```python
from build123d import *

# Parameters (mm, degrees)
SKETCH1_W                          = 8.4328
SKETCH1_H                          = 7.9375
F_5_16_24_TAPPED_HOLE1_D           = 7.9375
F_5_16_24_TAPPED_HOLE1_DEPTH       = 8.4328
F_5_16_24_TAPPED_HOLE1_CSINK_D     = 9.2075
F_5_16_24_TAPPED_HOLE1_CSINK_ANGLE = 120
SKETCH4_W                          = 18.873319712
SKETCH4_H                          = 3.5052
FILLET1_R                          = 0.254
F_6_32_TAPPED_HOLE1_D              = 3.5052
F_6_32_TAPPED_HOLE1_DEPTH          = 3.5062
CIRPATTERN1_COUNT                  = 4
CHAMFER1_SIZE                      = 0.635


with BuildPart() as part:
    # Sketch1 → Base-Revolve (revolve)
    with BuildSketch(Plane(origin=(0, 0, 0), x_dir=(0, 1, 0), z_dir=(0, 0, 1)), mode=Mode.PRIVATE) as base_revolve_sk:
        with Locations((-1.2446, 3.96875)):
            Rectangle(SKETCH1_W, SKETCH1_H)
    revolve(base_revolve_sk.sketch.rotate(Axis((0, -5.461, 0), (0, 1, 0)), 180), axis=Axis((0, -5.461, 0), (0, 1, 0)))  # turned: the seam where the file's is

    # 5_16-24 Tapped Hole1
    with Locations(Plane(origin=(0, 2.9718, 0), x_dir=(-1, 0, 0), z_dir=(0, 1, 0))):
        with Locations((0, 0)):
            CounterSinkHole(F_5_16_24_TAPPED_HOLE1_D / 2, F_5_16_24_TAPPED_HOLE1_CSINK_D / 2, depth=F_5_16_24_TAPPED_HOLE1_DEPTH, counter_sink_angle=F_5_16_24_TAPPED_HOLE1_CSINK_ANGLE)

    # Sketch4 → Revolve1 (revolve)
    with BuildSketch(Plane.XY, mode=Mode.PRIVATE) as revolve1_sk:
        with Locations((-9.436659856, -7.2136)):
            Rectangle(SKETCH4_W, SKETCH4_H)
    revolve(revolve1_sk.sketch.rotate(Axis((0, -29.193959905, 0), (0, 1, 0)), 180), axis=Axis((0, -29.193959905, 0), (0, 1, 0)))  # turned: the seam where the file's is

    # Sketch5 → 5_16-18 Tapped Hole2 (revolve, cut)
    with BuildSketch(Plane(origin=(0, -5.461, 0), x_dir=(0, 0, 1), z_dir=(1, 0, 0))):
        Polygon((0, 0), (0, 3.5052), (4.60375, 3.5052), (3.96875, 3.138582579), (3.96875, 0), align=None)
    revolve(axis=Axis((0, 0.889, 0), (0, -1, 0)), mode=Mode.SUBTRACT)

    # Fillet1
    fillet1_edges = [part.edges().sort_by_distance(p)[0] for p in [
        (-7.9375, -5.461, 0),
    ]]
    fillet(fillet1_edges, radius=FILLET1_R)

    # 6-32 Tapped Hole1
    with Locations(Plane.XZ.offset(8.9662)):
        with Locations((0, 12.7)):
            f_6_32_tapped_hole1 = Hole(F_6_32_TAPPED_HOLE1_D / 2, depth=F_6_32_TAPPED_HOLE1_DEPTH)

    # CirPattern1: 6-32 Tapped Hole1 ×4 about axis
    cirpattern1_axis = Axis((0, 0, 0), (0, 1, 0))
    for i in range(1, CIRPATTERN1_COUNT):
        add(f_6_32_tapped_hole1.rotate(cirpattern1_axis, i * 360 / CIRPATTERN1_COUNT), mode=Mode.SUBTRACT)

    # Chamfer1
    chamfer1_edges = [part.edges().sort_by_distance(p)[0] for p in [
        (-18.873319712, -5.461, 0),
    ]]
    chamfer(chamfer1_edges, length=CHAMFER1_SIZE)


solid = part.part
```
The listing builds one solid part. Answer for the finished solid, in the listing's coordinates (mm). A direction names the side the tool comes from. Give positions to 0.01 mm unless a question says otherwise; leave off trailing zeros. Order: outer loops, then holes, each group sorted by start corner. A loop starts at its lowest first (then second) coordinate and runs counter-clockwise, first axis right, second up. Notation, with made-up numbers: (88, 27.5) - (135, 27.5) arc R15 ccw to (135, 37.5) - close; hole circle Ø2 at (26, 85). An arc over 180 degrees is marked (long way). Answer in a Markdown table with one row per item. Add a question column.
Q1. Given P1, Ø5, axis at y = -7.5, z = -4, coming from the -X side; P2, Ø1, axis at x = 8, y = -7, coming from the +Z side; P3, Ø5.5, axis at x = 0, z = -12.7, coming from the +Y side, each flat-ended and moving along its own axis, determine where each tip first touches the part or whether it passes through.
Q2. The part is cut by section D-D (y = -3.5). Determine the outline of the cut face in (x, z) (1 decimal).
Q3. Find the intervals of material crossed by line 1 along Z through (x, y) = (0, -7); line 2 along Z through (x, y) = (0, 1); line 3 along Y through (x, z) = (7, -6.5), in increasing order. Write a range as [from, to].
Q4. The part is cut by section A-A (x = 0). Determine the outline of the cut face in (y, z), then the cut area to 3 significant figures.
Q5. For a pull along Z with two mould halves and no side action, classify faces 1 (the cylindrical face through (0.38, -7.19, 10.99)), 2 (the flat face through (4, -8.966, 4)), 3 (the cylindrical face through (-2.457, -7.511, -18.713)), 4 (the cylindrical face through (10.99, -7.19, -0.38)) as released by +Z, released by -Z, zero draft, split by the parting line, or undercut.
Q6. The part is cut by section C-C (y = -7.5). Determine the outline of the cut face in (x, z), then the cut area to 3 significant figures.
Q7. Which of the six approach directions +Z, -Z, +X, -X, +Y, -Y give full straight-line access (tool end or side, diameter ignored) to faces 5 (the cylindrical face through (-0.38, -7.19, -10.99)), 6 (the cylindrical face through (-1.72, -1.06, 7.75))?
Q8. The part is cut by section B-B (z = 0). Determine the outline of the cut face in (x, y), then the cut area to 3 significant figures.
Determined:
| question | item | result |
|---|---|---|
| 1 | P1 | stops at x = -18.81 |
| 1 | P2 | stops at z = 17.32 |
| 1 | P3 | stops at y = -5.46 |
| 2 | outline | circle Ø15.9 at (0, 0); hole circle Ø7.9 at (0, 0) |
| 3 | line 1 | z = [-18.87, -14.45], [-10.95, -3.97], [3.97, 10.95], [14.45, 18.87] |
| 3 | line 2 | z = [-7.94, -3.97], [3.97, 7.94] |
| 3 | line 3 | y = [-8.97, -5.46] |
| 4 | outline | (-8.97, -18.87) - (-6.1, -18.87) - (-5.46, -18.24) - (-5.46, -14.45) - (-8.97, -14.45) - close; (-8.97, -10.95) - (-5.46, -10.95) - (-5.46, -8.19) arc R0.25 cw to (-5.21, -7.94) - (2.97, -7.94) - (2.97, -4.6) - (2.61, -3.97) - (-8.6, -3.97) - (-8.97, -4.6) - close; (-8.97, 4.6) - (-8.6, 3.97) - (2.61, 3.97) - (2.97, 4.6) - (2.97, 7.94) - (-5.21, 7.94) arc R0.25 cw to (-5.46, 8.19) - (-5.46, 10.95) - (-8.97, 10.95) - close; (-8.97, 14.45) - (-5.46, 14.45) - (-5.46, 18.24) - (-6.1, 18.87) - (-8.97, 18.87) - close |
| 4 | area | 146 mm² |
| 5 | face 1 | undercut |
| 5 | face 2 | zero draft |
| 5 | face 3 | split by the parting line |
| 5 | face 4 | undercut |
| 6 | outline | circle Ø37.75 at (0, 0); hole circle Ø3.51 at (-12.7, 0); hole circle Ø7.94 at (0, 0); hole circle Ø3.51 at (0, -12.7); hole circle Ø3.51 at (0, 12.7); hole circle Ø3.51 at (12.7, 0) |
| 6 | area | 1,030 mm² |
| 7 | face 5 | +Y, -Y |
| 7 | face 6 | +Y |
| 8 | outline | (-18.87, -8.97) - (-14.45, -8.97) - (-14.45, -5.46) - (-18.24, -5.46) - (-18.87, -6.1) - close; (-10.95, -8.97) - (-4.6, -8.97) - (-3.97, -8.6) - (-3.97, 2.61) - (-4.6, 2.97) - (-7.94, 2.97) - (-7.94, -5.21) arc R0.25 cw to (-8.19, -5.46) - (-10.95, -5.46) - close; (3.97, -8.6) - (4.6, -8.97) - (10.95, -8.97) - (10.95, -5.46) - (8.19, -5.46) arc R0.25 cw to (7.94, -5.21) - (7.94, 2.97) - (4.6, 2.97) - (3.97, 2.61) - close; (14.45, -8.97) - (18.87, -8.97) - (18.87, -6.1) - (18.24, -5.46) - (14.45, -5.46) - close |
| 8 | area | 146 mm² |
